Can you work these out from the model? Positions are in its coordinate system, mm. A direction names the side the tool comes from. Give positions to 0.01 mm unless a question says otherwise; leave off trailing zeros. Use CSV: the item, a comma, the result in double quotes.
from build123d import *

# Parameters (mm, degrees)
F1_DEPTH = 2
F2_DEPTH = 2
F4_DEPTH = 2


with BuildPart() as f1:
    # F0 (on Top) → F1 (new body)
    with BuildSketch(Plane.XY):
        with BuildLine():
            ThreePointArc((24.235519, -6.135113), (20.423062, -1.358402), (24.834565, 2.871307))
            ThreePointArc((24.834565, 2.871307), (24.40188, 5.435831), (23.705109, 7.941526))
            ThreePointArc((23.705109, 7.941526), (17.91538, 9.89878), (19.33982, 15.842076))
            ThreePointArc((19.33982, 15.842076), (17.589336, 17.765564), (15.648493, 19.496786))
            ThreePointArc((15.648493, 19.496786), (9.719693, 18.01317), (7.704819, 23.783098))
            ThreePointArc((7.704819, 23.783098), (5.192302, 24.454856), (2.623592, 24.861954))
            ThreePointArc((2.623592, 24.861954), (-1.561929, 20.408505), (-6.376408, 24.173155))
            ThreePointArc((-6.376408, 24.173155), (-8.853251, 23.379905), (-11.234281, 22.333628))
            ThreePointArc((-11.234281, 22.333628), (-12.347649, 16.324284), (-18.43317, 16.888406))
            ThreePointArc((-18.43317, 16.888406), (-20.08796, 14.881998), (-21.525349, 12.714532))
            ThreePointArc((-21.525349, 12.714532), (-19.213078, 7.057219), (-24.637531, 4.241707))
            ThreePointArc((-24.637531, 4.241707), (-24.944883, 1.659163), (-24.982271, -0.941337))
            ThreePointArc((-24.982271, -0.941337), (-19.97849, -4.450464), (-23.01965, -9.751704))
            ThreePointArc((-23.01965, -9.751704), (-21.881982, -12.090445), (-20.507499, -14.298339))
            ThreePointArc((-20.507499, -14.298339), (-14.400873, -14.545156), (-14.093192, -20.649018))
            ThreePointArc((-14.093192, -20.649018), (-11.871706, -22.001422), (-9.52174, -23.115719))
            ThreePointArc((-9.52174, -23.115719), (-4.25108, -20.021864), (-0.692246, -24.990414))
            ThreePointArc((-0.692246, -24.990414), (1.907752, -24.927103), (4.487104, -24.594022))
            ThreePointArc((4.487104, -24.594022), (7.2484, -19.141771), (12.928483, -21.397531))
            ThreePointArc((12.928483, -21.397531), (15.081513, -19.938605), (17.071324, -18.263896))
            ThreePointArc((17.071324, -18.263896), (16.446565, -12.184301), (22.444511, -11.011082))
            ThreePointArc((22.444511, -11.011082), (23.467, -8.619741), (24.235519, -6.135113))
        make_face()
        with BuildLine():
            ThreePointArc((9.357447, 3.52678), (9.83805, 1.792418), (10, 0))
            ThreePointArc((10, 0), (9.999547, -0.095211), (9.998187, -0.190414))
            ThreePointArc((9.998187, -0.190414), (9.958528, -0.909789), (9.867177, -1.624442))
            ThreePointArc((9.867177, -1.624442), (9.383729, -3.456246), (8.563477, -5.163997))
            ThreePointArc((8.563477, -5.163997), (8.169444, -5.767165), (7.733005, -6.340397))
            ThreePointArc((7.733005, -6.340397), (6.398425, -7.685061), (4.83419, -8.753891))
            ThreePointArc((4.83419, -8.753891), (4.191363, -9.079233), (3.52678, -9.357447))
            ThreePointArc((3.52678, -9.357447), (1.698668, -9.85467), (-0.190414, -9.998187))
            ThreePointArc((-0.190414, -9.998187), (-0.909789, -9.958528), (-1.624442, -9.867177))
            ThreePointArc((-1.624442, -9.867177), (-3.456246, -9.383729), (-5.163997, -8.563477))
            ThreePointArc((-5.163997, -8.563477), (-5.767165, -8.169444), (-6.340397, -7.733005))
            ThreePointArc((-6.340397, -7.733005), (-7.685061, -6.398425), (-8.753891, -4.83419))
            ThreePointArc((-8.753891, -4.83419), (-9.079233, -4.191363), (-9.357447, -3.52678))
            ThreePointArc((-9.357447, -3.52678), (-9.85467, -1.698668), (-9.998187, 0.190414))
            ThreePointArc((-9.998187, 0.190414), (-9.958528, 0.909789), (-9.867177, 1.624442))
            ThreePointArc((-9.867177, 1.624442), (-9.383729, 3.456246), (-8.563477, 5.163997))
            ThreePointArc((-8.563477, 5.163997), (-8.169444, 5.767165), (-7.733005, 6.340397))
            ThreePointArc((-7.733005, 6.340397), (-6.398425, 7.685061), (-4.83419, 8.753891))
            ThreePointArc((-4.83419, 8.753891), (-4.191363, 9.079233), (-3.52678, 9.357447))
            ThreePointArc((-3.52678, 9.357447), (-1.698668, 9.85467), (0.190414, 9.998187))
            ThreePointArc((0.190414, 9.998187), (0.909789, 9.958528), (1.624442, 9.867177))
            ThreePointArc((1.624442, 9.867177), (3.456246, 9.383729), (5.163997, 8.563477))
            ThreePointArc((5.163997, 8.563477), (5.767165, 8.169444), (6.340397, 7.733005))
            ThreePointArc((6.340397, 7.733005), (7.685061, 6.398425), (8.753891, 4.83419))
            ThreePointArc((8.753891, 4.83419), (9.079233, 4.191363), (9.357447, 3.52678))
        make_face(mode=Mode.SUBTRACT)
    extrude(amount=F1_DEPTH)

    # F0 (on Top) → F2 (join)
    with BuildSketch(Plane.XY):
        with BuildLine():
            Line((7.95383, 2.997763), (9.357447, 3.52678))
            ThreePointArc((9.357447, 3.52678), (9.079233, 4.191363), (8.753891, 4.83419))
            Line((8.753891, 4.83419), (7.440807, 4.109062))
            ThreePointArc((7.440807, 4.109062), (7.717348, 3.562659), (7.95383, 2.997763))
        make_face()
        with BuildLine():
            Line((5.389337, 6.573054), (6.340397, 7.733005))
            ThreePointArc((6.340397, 7.733005), (5.767165, 8.169444), (5.163997, 8.563477))
            Line((5.163997, 8.563477), (4.389397, 7.278955))
            ThreePointArc((4.389397, 7.278955), (4.90209, 6.944027), (5.389337, 6.573054))
        make_face()
        with BuildLine():
            Line((1.380776, 8.387101), (1.624442, 9.867177))
            ThreePointArc((1.624442, 9.867177), (0.909789, 9.958528), (0.190414, 9.998187))
            Line((0.190414, 9.998187), (0.161852, 8.498459))
            ThreePointArc((0.161852, 8.498459), (0.773321, 8.464749), (1.380776, 8.387101))
        make_face()
        with BuildLine():
            ThreePointArc((9.867177, -1.624442), (9.958528, -0.909789), (9.998187, -0.190414))
            Line((9.998187, -0.190414), (8.498459, -0.161852))
            ThreePointArc((8.498459, -0.161852), (8.464749, -0.773321), (8.387101, -1.380776))
            Line((8.387101, -1.380776), (9.867177, -1.624442))
        make_face()
        with BuildLine():
            ThreePointArc((7.733005, -6.340397), (8.169444, -5.767165), (8.563477, -5.163997))
            Line((8.563477, -5.163997), (7.278955, -4.389397))
            ThreePointArc((7.278955, -4.389397), (6.944027, -4.90209), (6.573054, -5.389337))
            Line((6.573054, -5.389337), (7.733005, -6.340397))
        make_face()
        with BuildLine():
            ThreePointArc((3.52678, -9.357447), (4.191363, -9.079233), (4.83419, -8.753891))
            Line((4.83419, -8.753891), (4.109062, -7.440807))
            ThreePointArc((4.109062, -7.440807), (3.562659, -7.717348), (2.997763, -7.95383))
            Line((2.997763, -7.95383), (3.52678, -9.357447))
        make_face()
        with BuildLine():
            ThreePointArc((-1.624442, -9.867177), (-0.909789, -9.958528), (-0.190414, -9.998187))
            Line((-0.190414, -9.998187), (-0.161852, -8.498459))
            ThreePointArc((-0.161852, -8.498459), (-0.773321, -8.464749), (-1.380776, -8.387101))
            Line((-1.380776, -8.387101), (-1.624442, -9.867177))
        make_face()
        with BuildLine():
            ThreePointArc((-6.340397, -7.733005), (-5.767165, -8.169444), (-5.163997, -8.563477))
            Line((-5.163997, -8.563477), (-4.389397, -7.278955))
            ThreePointArc((-4.389397, -7.278955), (-4.90209, -6.944027), (-5.389337, -6.573054))
            Line((-5.389337, -6.573054), (-6.340397, -7.733005))
        make_face()
        with BuildLine():
            ThreePointArc((-9.357447, -3.52678), (-9.079233, -4.191363), (-8.753891, -4.83419))
            Line((-8.753891, -4.83419), (-7.440807, -4.109062))
            ThreePointArc((-7.440807, -4.109062), (-7.717348, -3.562659), (-7.95383, -2.997763))
            Line((-7.95383, -2.997763), (-9.357447, -3.52678))
        make_face()
        with BuildLine():
            Line((-8.387101, 1.380776), (-9.867177, 1.624442))
            ThreePointArc((-9.867177, 1.624442), (-9.958528, 0.909789), (-9.998187, 0.190414))
            Line((-9.998187, 0.190414), (-8.498459, 0.161852))
            ThreePointArc((-8.498459, 0.161852), (-8.464749, 0.773321), (-8.387101, 1.380776))
        make_face()
        with BuildLine():
            Line((-6.573054, 5.389337), (-7.733005, 6.340397))
            ThreePointArc((-7.733005, 6.340397), (-8.169444, 5.767165), (-8.563477, 5.163997))
            Line((-8.563477, 5.163997), (-7.278955, 4.389397))
            ThreePointArc((-7.278955, 4.389397), (-6.944027, 4.90209), (-6.573054, 5.389337))
        make_face()
        with BuildLine():
            Line((-2.997763, 7.95383), (-3.52678, 9.357447))
            ThreePointArc((-3.52678, 9.357447), (-4.191363, 9.079233), (-4.83419, 8.753891))
            Line((-4.83419, 8.753891), (-4.109062, 7.440807))
            ThreePointArc((-4.109062, 7.440807), (-3.562659, 7.717348), (-2.997763, 7.95383))
        make_face()
    extrude(amount=F2_DEPTH)

    # F3 (on face) → F4 (cut)
    with BuildSketch(Plane.XY.offset(2)):
        with BuildLine():
            ThreePointArc((-11.920186, 6.882123), (-6.882123, 11.920186), (0, 13.764245))
            ThreePointArc((0, 13.764245), (2.5, 16.264245), (0, 18.764245))
            ThreePointArc((0, 18.764245), (-9.382123, 16.250313), (-16.250313, 9.382123))
            ThreePointArc((-16.250313, 9.382123), (-15.335249, 5.967059), (-11.920186, 6.882123))
        make_face()
        with BuildLine():
            ThreePointArc((0, -13.764245), (-6.882123, -11.920186), (-11.920186, -6.882123))
            ThreePointArc((-11.920186, -6.882123), (-15.335249, -5.967059), (-16.250313, -9.382123))
            ThreePointArc((-16.250313, -9.382123), (-9.382123, -16.250313), (0, -18.764245))
            ThreePointArc((0, -18.764245), (2.5, -16.264245), (0, -13.764245))
        make_face()
        with BuildLine():
            ThreePointArc((11.920186, 6.882123), (13.764245, 0), (11.920186, -6.882123))
            ThreePointArc((11.920186, -6.882123), (12.835249, -10.297186), (16.250313, -9.382123))
            ThreePointArc((16.250313, -9.382123), (18.764245, 0), (16.250313, 9.382123))
            ThreePointArc((16.250313, 9.382123), (12.835249, 10.297186), (11.920186, 6.882123))
        make_face()
    extrude(amount=-F4_DEPTH, mode=Mode.SUBTRACT)


solid = f1.part
Q1. For faces 4 (the cylindrical face through (20.418, -1.452, 0.986)), 5 (the cylindrical face through (18.764, -0.138, 1.014)), which set-ups out of +Z, -Z, +X, -X, +Y, -Y let a thin tool reach every point of the face, with its end or its side?
Model answer:
face 4,"+Z, -Z, +X"
face 5,"+Z, -Z"
Q2. If we mould it in two halves opening along Y, with no side actions, what happens to faces 1 (the flat face through (0, 11, 0)), 2 (the cylindrical face through (17.96, 9.82, 0.99)), 3 (the cylindrical face through (17.615, 17.74, 0.986))? For each: released by +Y, released by -Y, zero draft, split by the parting line, or undercut.
Model answer:
face 1,"zero draft"
face 2,"undercut"
face 3,"released by +Y"
Q3. I want a section at A-A, the plane z = 1.2. State how many separate pieces and enclosed holes the cut face has, then the cut area to 3 significant figures.
Model answer:
separate pieces,"1"
enclosed holes,"4"
area,"1,020 mm2"
Q4. Please list where these lines run through material, in increasing order: L1, parallel to Y at x = -6, z = 0.55; L2, parallel to X at y = 8, z = 1.5; L3, parallel to Y at x = -8, z = 1.85. Write a range as from..to.
Model answer:
L1,"-20..-17.78, -12.39..-7.32, 8..12.39, 17.78..22.98"
L2,"-18.98..-16.58, -11.2..-6, -4.42..-3.02, 4.82..11.59, 16.97..19.93"
L3,"-20.9..-16.97, -11.2..-6, -4.42..-3.02, 4.82..11.2, 16.97..23.69"
Q5. I'm going to push a flat-ended pin straight in: P1, Ø1, axis at x = -2.5, y = 8.5, coming from the -Z side. Where does the tip first touch, or does it pass through?
Model answer:
P1,"through"
